```python
from build123d import *

# Parameters (mm, degrees)
BOSS_EXTRUDE1_DEPTH = 6
SKETCH2_W           = 66
SKETCH2_H           = 415
BOSS_EXTRUDE2_DEPTH = 6
SKETCH3_R           = 10
CUT_EXTRUDE1_DEPTH  = 6


with BuildPart() as part:
    # Sketch1 → Boss-Extrude1 (new body)
    with BuildSketch(Plane.XY):
        Polygon((23, 395), (23, 0), (43, 0), (43, 415), (-23, 415), (-23, 395), align=None)
    extrude(amount=-BOSS_EXTRUDE1_DEPTH)

    # Sketch2 → Boss-Extrude2 (add)
    with BuildSketch(Plane.XY):
        with Locations((10, 207.5)):
            Rectangle(SKETCH2_W, SKETCH2_H)
    extrude(amount=BOSS_EXTRUDE2_DEPTH)

    # Sketch3 → Cut-Extrude1 (cut)
    with BuildSketch(Plane(origin=(0, 0, -6), x_dir=(-1, 0, 0), z_dir=(0, 0, -1))):
        with Locations((-23, 395)):
            Circle(SKETCH3_R)
    extrude(amount=-CUT_EXTRUDE1_DEPTH, mode=Mode.SUBTRACT)


solid = part.part
```
Geometry: final body of the model. Coordinates: model frame, mm. Give positions to 0.01 mm unless a question says otherwise; leave off trailing zeros. Order: outer loops, then holes, each group sorted by start corner. A loop starts at its lowest first (then second) coordinate and runs counter-clockwise, first axis right, second up. Notation, with made-up numbers: M 76.25,53 L 89.25,53 A28 ccw 89.25,78 Z; hole C -28.5,31 d9. An arc over 180 degrees is marked long. Answer as CSV lines item,"result". Start each with the question number.
1) Line query: line 1 (Z direction, x = 10, y = 195); line 2 (Y direction, x = 8.5, z = -4.5); line 3 (X direction, y = 112, z = -4.25). Output: solid intervals per line, ascending. Write a range as from..to.
2) Cut plane A-A (x = -9). Output: boundary loops of the cut face in (y, z).
3) Mould query, pull axis X, two halves, no side actions, for faces 1 (the flat face through (-23, 205, 4)), 2 (the cylindrical face through (29.834, 402.3, -3.042)), 3 (the flat face through (10, 210, 6)). Classes: +X half, -X half, draft (parallel to the pull), parting line (faces both ways), or undercut.
4) Cut plane C-C (x = 29). Output: boundary loops of the cut face in (y, z), then the cut area to 3 significant figures.
5) First-contact query: P1, Ø3, axis at y = 232, z = -4, coming from the -X side; P2, Ø5, axis at x = 6.5, y = 129.5, coming from the -Z side; P3, Ø4, axis at x = -4, z = 3, coming from the -Y side; P4, Ø4, axis at x = -0.5, z = -2.5, coming from the -Y side. Flat tips, straight axial feed; report the tip coordinate or a pass-through.
6) Cut plane B-B (y = 150.5). Output: boundary loops of the cut face in (x, z), then the cut area to 3 significant figures.
Findings below:
1,line 1,"z = 0..6"
1,line 2,"y = 395..415"
1,line 3,"x = 23..43"
2,outline,"M 0,0 L 395,0 L 395,-6 L 415,-6 L 415,6 L 0,6 Z"
3,face 1,"-X half"
3,face 2,"undercut"
3,face 3,"draft"
4,outline,"M 0,-6 L 387,-6 L 387,0 L 403,0 L 403,-6 L 415,-6 L 415,6 L 0,6 Z"
4,area,"4,880 mm²"
5,P1,"stops at x = 23"
5,P2,"stops at z = 0"
5,P3,"stops at y = 0"
5,P4,"stops at y = 395"
6,outline,"M -23,0 L 23,0 L 23,-6 L 43,-6 L 43,6 L -23,6 Z"
6,area,"516 mm²"
